Can you work these out from the model? Positions are in its coordinate system, mm. A direction names the side the tool comes from. Coordinates: 2 decimals unless noted, no trailing zeros. Write each loop counter-clockwise with the first axis right and the second up, starting at its lowest first coordinate (ties: lowest second). Pieces come first, ordered by that corner, then holes. Notation, with made-up numbers: M 55.5,-20.5 L 70.5,-20.5 A18 ccw 70.5,14.5 Z; hole C 63,20 d4. An arc over 180 degrees is marked long. Answer as a JSON object with one key per item and string values. Group by question number.
from build123d import *

# Parameters (mm, degrees)
F0_W     = 83
F0_H     = 7.6
F0_W_2   = 78
F0_H_2   = 2.6
F1_DEPTH = 8
F2_W     = 83
F2_H     = 7.6
F2_W_2   = 78
F2_H_2   = 2.6
F3_DEPTH = 3.5
F4_W     = 3
F4_H     = 3
F4_W_2   = 4.2
F4_H_2   = 4.2
F4_W_3   = 11
F5_DEPTH = 6


with BuildPart() as f1:
    # F0 (on Front) → F1 (new body)
    with BuildSketch(Plane.XZ):
        Rectangle(F0_W, F0_H)
        Rectangle(F0_W_2, F0_H_2, mode=Mode.SUBTRACT)
    extrude(amount=F1_DEPTH)

    # F2 (on face) → F3 (join)
    with BuildSketch(Plane.XZ.offset(8)):
        Rectangle(F2_W, F2_H)
        Rectangle(F2_W_2, F2_H_2, mode=Mode.SUBTRACT)
        Rectangle(F2_W_2, F2_H_2)
    extrude(amount=F3_DEPTH)

    # F4 (on face) → F5 (join)
    with BuildSketch(Plane.XY.offset(3.8)):
        with Locations((-40, -10)):
            Rectangle(F4_W, F4_H)
        with Locations((-36.4, -10)):
            Rectangle(F4_W_2, F4_H)
        with Locations((-40, -6.4)):
            Rectangle(F4_W, F4_H_2)
        with Locations((-32.8, -10)):
            Rectangle(F4_W, F4_H)
        with Locations((-40, -2.8)):
            Rectangle(F4_W, F4_H)
        with Locations((-29.2, -10)):
            Rectangle(F4_W_2, F4_H)
        with Locations((-32.8, -6.4)):
            Rectangle(F4_W, F4_H_2)
        with Locations((-36.4, -2.8)):
            Rectangle(F4_W_2, F4_H)
        with Locations((-25.6, -10)):
            Rectangle(F4_W, F4_H)
        with Locations((-32.8, -2.8)):
            Rectangle(F4_W, F4_H)
        with Locations((-22, -10)):
            Rectangle(F4_W_2, F4_H)
        with Locations((-25.6, -6.4)):
            Rectangle(F4_W, F4_H_2)
        with Locations((-29.2, -2.8)):
            Rectangle(F4_W_2, F4_H)
        with Locations((-18.4, -10)):
            Rectangle(F4_W, F4_H)
        with Locations((-25.6, -2.8)):
            Rectangle(F4_W, F4_H)
        with Locations((40, -2.8)):
            Rectangle(F4_W, F4_H)
        with Locations((-14.8, -10)):
            Rectangle(F4_W_2, F4_H)
        with Locations((-18.4, -6.4)):
            Rectangle(F4_W, F4_H_2)
        with Locations((-22, -2.8)):
            Rectangle(F4_W_2, F4_H)
        with Locations((36.4, -2.8)):
            Rectangle(F4_W_2, F4_H)
        with Locations((40, -6.4)):
            Rectangle(F4_W, F4_H_2)
        with Locations((-11.2, -10)):
            Rectangle(F4_W, F4_H)
        with Locations((-18.4, -2.8)):
            Rectangle(F4_W, F4_H)
        with Locations((32.8, -2.8)):
            Rectangle(F4_W, F4_H)
        with Locations((40, -10)):
            Rectangle(F4_W, F4_H)
        with Locations((-7.6, -10)):
            Rectangle(F4_W_2, F4_H)
        with Locations((-11.2, -6.4)):
            Rectangle(F4_W, F4_H_2)
        with Locations((-14.8, -2.8)):
            Rectangle(F4_W_2, F4_H)
        with Locations((29.2, -2.8)):
            Rectangle(F4_W_2, F4_H)
        with Locations((32.8, -6.4)):
            Rectangle(F4_W, F4_H_2)
        with Locations((36.4, -10)):
            Rectangle(F4_W_2, F4_H)
        with Locations((0, -10)):
            Rectangle(F4_W_3, F4_H)
        with Locations((-11.2, -2.8)):
            Rectangle(F4_W, F4_H)
        with Locations((25.6, -2.8)):
            Rectangle(F4_W, F4_H)
        with Locations((32.8, -10)):
            Rectangle(F4_W, F4_H)
        with Locations((7.6, -10)):
            Rectangle(F4_W_2, F4_H)
        with Locations((0, -6.4)):
            Rectangle(F4_W_3, F4_H_2)
        with Locations((-7.6, -2.8)):
            Rectangle(F4_W_2, F4_H)
        with Locations((22, -2.8)):
            Rectangle(F4_W_2, F4_H)
        with Locations((25.6, -6.4)):
            Rectangle(F4_W, F4_H_2)
        with Locations((29.2, -10)):
            Rectangle(F4_W_2, F4_H)
        with Locations((11.2, -10)):
            Rectangle(F4_W, F4_H)
        with Locations((0, -2.8)):
            Rectangle(F4_W_3, F4_H)
        with Locations((18.4, -2.8)):
            Rectangle(F4_W, F4_H)
        with Locations((25.6, -10)):
            Rectangle(F4_W, F4_H)
        with Locations((14.8, -10)):
            Rectangle(F4_W_2, F4_H)
        with Locations((11.2, -6.4)):
            Rectangle(F4_W, F4_H_2)
        with Locations((7.6, -2.8)):
            Rectangle(F4_W_2, F4_H)
        with Locations((14.8, -2.8)):
            Rectangle(F4_W_2, F4_H)
        with Locations((18.4, -6.4)):
            Rectangle(F4_W, F4_H_2)
        with Locations((22, -10)):
            Rectangle(F4_W_2, F4_H)
        with Locations((18.4, -10)):
            Rectangle(F4_W, F4_H)
        with Locations((11.2, -2.8)):
            Rectangle(F4_W, F4_H)
    extrude(amount=F5_DEPTH)


solid = f1.part
Q1. If we section it at C-C on z = 4.5: Give the number of separate pieces and of enclosed holes in the cut face, and give its area (3 significant figures).
Q2. If we section it at A-A on y = -3: List the corners of the cut face in (x, z) for me.
Q3. If we section it at D-D on z = -0.25: List the corners of the cut face in (x, y) for me.
Q4. We'd pull the mould along X, two halves only. Please class faces 4 (the flat face through (-1, -11.5, 3)), 5 (the flat face through (-12.7, -6, 7)), 6 (the flat face through (-41.5, -6, 3)): pulls with the +X half, pulls with the -X half, needs draft (parallel to the pull), parting line crosses it, or undercut.
Q5. On a 3-axis mill with a long thin cutter (end or side, diameter ignored), from which of +Z, -Z, +X, -X, +Y, -Y can I reach the whole of each face in a straight line? I mean faces 1 (the flat face through (-1, -6, -3.8)), 2 (the flat face through (39, -4, 0)), 3 (the flat face through (-15, -4.3, 7)). Say none if no direction works.
Q6. Will these pins go through, and if not, where does the flat tip stop? pin 1 (2 mm diameter, centred on x = -36.5, y = -6.5, fed in from +Z); pin 2 (3.5 mm diameter, centred on x = 30, z = 6.5, fed in from +Y).
Q7. Please list where these lines run through material, in increasing order: L1, parallel to Z at x = 36, y = -5; L2, parallel to Z at x = -34, y = -5.25; L3, parallel to X at y = -7.25, z = 1.25.
Q8. If we section it at B-B on x = 21.5: List the corners of the cut face in (y, z) for me.
Reply:
{
 "1": {"separate pieces": "1", "enclosed holes": "10", "area": "670 mm^2"},
 "2": {"outline": "M -41.5,-3.8 L 41.5,-3.8 L 41.5,9.8 L -41.5,9.8 Z; hole M -39,-1.3 L 39,-1.3 L 39,1.3 L -39,1.3 Z"},
 "3": {"outline": "M -41.5,-11.5 L 41.5,-11.5 L 41.5,0 L 39,0 L 39,-8 L -39,-8 L -39,0 L -41.5,0 Z"},
 "4": {"face 4": "needs draft", "face 5": "undercut", "face 6": "pulls with the -X half"},
 "5": {"face 1": "-Z, +X, -X, +Y, -Y", "face 2": "+Y", "face 3": "+Z"},
 "6": {"pin 1": "z = 3.8", "pin 2": "y = -1.3"},
 "7": {"L1": "-3.8 to -1.3, 1.3 to 3.8", "L2": "-3.8 to -1.3, 1.3 to 9.8", "L3": "-41.5 to -39, 39 to 41.5"},
 "8": {"outline": "M -11.5,-3.8 L 0,-3.8 L 0,-1.3 L -8,-1.3 L -8,1.3 L 0,1.3 L 0,3.8 L -1.3,3.8 L -1.3,9.8 L -4.3,9.8 L -4.3,3.8 L -8.5,3.8 L -8.5,9.8 L -11.5,9.8 Z"}
}
